from build123d import *

# Parameters (mm, degrees)
SKETCH_1_R      = 1.5
EXTRUDE_1_DEPTH = 1


with BuildPart() as part:
    # 草图1 → 凸台-拉伸1 (new body)
    with BuildSketch(Plane(origin=(0, 0, 0), x_dir=(1, 0, 0), z_dir=(0, 1, 0))):
        with BuildLine():
            ThreePointArc((89.399493256, 56.953758485), (0, 106), (-89.399493256, 56.953758485))
            ThreePointArc((-89.399493256, 56.953758485), (-88.175125906, 51.430994268), (-82.65236169, 52.655361618))
            ThreePointArc((-82.65236169, 52.655361618), (0, 98), (82.65236169, 52.655361618))
            ThreePointArc((82.65236169, 52.655361618), (88.175125906, 51.430994268), (89.399493256, 56.953758485))
        make_face()
        with Locations(Location((0, 102, 0), (0, 0, 270))):
            Circle(SKETCH_1_R, mode=Mode.SUBTRACT)
        with Locations(Location((-86.025927473, 54.804560051, 0), (0, 0, 270))):
            Circle(SKETCH_1_R, mode=Mode.SUBTRACT)
        with Locations(Location((86.025927473, 54.804560051, 0), (0, 0, 270))):
            Circle(SKETCH_1_R, mode=Mode.SUBTRACT)
        with BuildLine():
            ThreePointArc((-8.078431373, 102.682710066), (-49.544575655, 90.301356707), (-82.264932334, 61.979681413))
            ThreePointArc((-82.264932334, 61.979681413), (-82.067988151, 60.579248269), (-80.667555008, 60.776192453))
            ThreePointArc((-80.667555008, 60.776192453), (-48.58254506, 88.547932305), (-7.921568627, 100.688871036))
            ThreePointArc((-7.921568627, 100.688871036), (-7.003080485, 101.764221924), (-8.078431373, 102.682710066))
        make_face(mode=Mode.SUBTRACT)
        with BuildLine():
            ThreePointArc((82.264932334, 61.979681413), (49.544575655, 90.301356707), (8.078431373, 102.682710066))
            ThreePointArc((8.078431373, 102.682710066), (7.003080485, 101.764221924), (7.921568627, 100.688871036))
            ThreePointArc((7.921568627, 100.688871036), (48.58254506, 88.547932305), (80.667555008, 60.776192453))
            ThreePointArc((80.667555008, 60.776192453), (82.067988151, 60.579248269), (82.264932334, 61.979681413))
        make_face(mode=Mode.SUBTRACT)
    extrude(amount=EXTRUDE_1_DEPTH)


solid = part.part
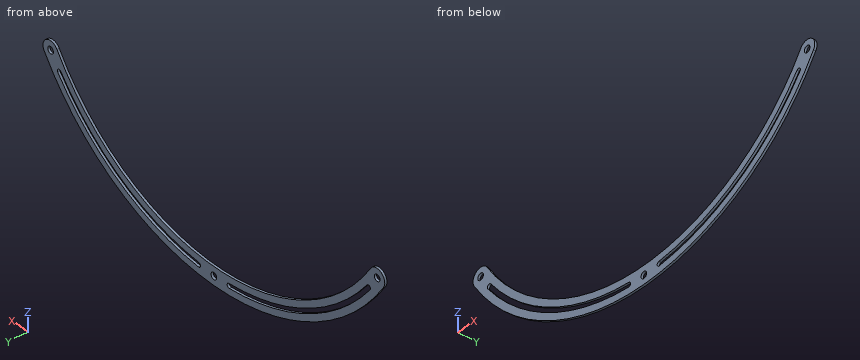
Can you work these out from the model? Positions are in its coordinate system, mm. Coordinates: 2 decimals unless noted, no trailing zeros. Write each loop counter-clockwise with the first axis right and the second up, starting at its lowest first coordinate (ties: lowest second). Pieces come first, ordered by that corner, then holes. Notation, with made-up numbers: (-39.5, -5) -> (18.5, -5) arc R6 ccw to (18.5, 4) -> close; hole circle Ø1 at (30, -21.5). An arc over 180 degrees is marked (long way). Write each question's results on one line, items separated by ' | '. Start each with the question number.
Q1. Imagine slicing it at A-A (x = 36.5). Write out the boundary of the cut face in (y, z), then the cut area to 3 significant figures.
Q2. If I drill on probe 1 along X at (y, z) = (0.2, -86); probe 2 along X at (y, z) = (0.2, -55.5) (3 decimals); probe 3 along Z at (x, y) = (57, 0.4), over which ranges is the centre line in solid material (lowest first)?
Q3. I'm going to push a flat-ended pin straight in: pin 1 (3.5 mm diameter, centred on x = 86.03, z = -54.8, fed in from -Y). Where does the tip first touch, or does it pass through?
Q4. Imagine slicing it at D-D (x = 13). Write out the boundary of the cut face in (y, z), then the cut area to 3 significant figures.
Q5. Imagine slicing it at C-C (y = 0.35). Write out the boundary of the cut face in (x, z), then the cut area to 3 significant figures.
Q6. Imagine slicing it at B-B (z = -71). Write out the boundary of the cut face in (x, y), then the cut area to 3 significant figures.
Taken from the geometry:
1) outline: (0, -99.52) -> (1, -99.52) -> (1, -96.32) -> (0, -96.32) -> close; (0, -94.17) -> (1, -94.17) -> (1, -90.95) -> (0, -90.95) -> close | area: 6.43 mm^2
2) probe 1: x = -61.97 to -56.68, -52.96 to -46.99, 46.99 to 52.96, 56.68 to 61.97 | probe 2: x = -89.965 to -87.355, -84.697 to -80.77, 80.77 to 84.697, 87.355 to 89.965 | probe 3: z = -89.37 to -85.79, -83.38 to -79.72
3) pin 1: stops at y = 0
4) outline: (0, -105.2) -> (1, -105.2) -> (1, -102.18) -> (0, -102.18) -> close; (0, -100.16) -> (1, -100.16) -> (1, -97.13) -> (0, -97.13) -> close | area: 6.05 mm^2
5) outline: (-89.4, -56.95) arc R106 ccw to (89.4, -56.95) arc R4 ccw to (82.65, -52.66) arc R98 cw to (-82.65, -52.66) arc R4 ccw to start; hole circle Ø3 at (-86.03, -54.8); hole (-82.26, -61.98) arc R103 ccw to (-8.08, -102.68) arc R1 ccw to (-7.92, -100.69) arc R101 cw to (-80.67, -60.78) arc R1 ccw to start; hole circle Ø3 at (0, -102); hole (7.92, -100.69) arc R1 ccw to (8.08, -102.68) arc R103 ccw to (82.26, -61.98) arc R1 ccw to (80.67, -60.78) arc R101 cw to start; hole circle Ø3 at (86.03, -54.8) | area: 1,320 mm^2
6) outline: (-78.71, 0) -> (-74.62, 0) -> (-74.62, 1) -> (-78.71, 1) -> close; (-71.83, 0) -> (-67.55, 0) -> (-67.55, 1) -> (-71.83, 1) -> close; (67.55, 0) -> (71.83, 0) -> (71.83, 1) -> (67.55, 1) -> close; (74.62, 0) -> (78.71, 0) -> (78.71, 1) -> (74.62, 1) -> close | area: 16.7 mm^2
